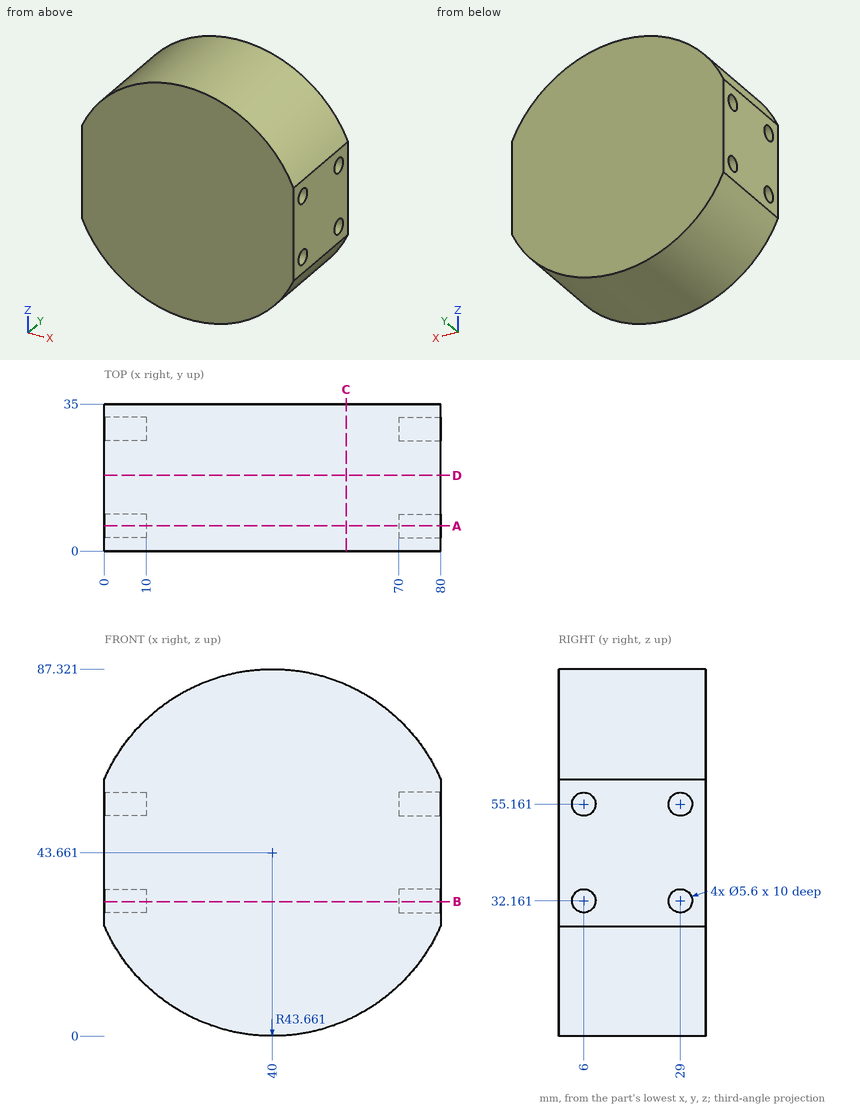
For this review, use the dimensioned drawing (mm, ordinates from the lowest corner) and the shaded views. Coordinates: 2 decimals unless noted, no trailing zeros. Order: outer loops, then holes, each group sorted by start corner. A loop starts at its lowest first (then second) coordinate and runs counter-clockwise, first axis right, second up. Notation, with made-up numbers: M 13,85 L 57,85 A13 ccw 57,105 Z; hole C 56,-13 d8. An arc over 180 degrees is marked long. Answer as a JSON object with one key per item and string values. Group by question number.
1) Add section B-B, the plane z = 32. Write out the cut boundary in (x, y) (1 decimal).
2) For pin 1 (5 mm diameter, centred on y = 6, z = 55.16, fed in from +X); pin 2 (6 mm diameter, centred on x = 68, y = 25, fed in from +Z) (1 decimal); pin 3 (2 mm diameter, centred on x = 59.5, y = 8.5, fed in from +Z), all flat-tipped, find the tip position at first contact; note any pin that passes through.
3) Add section D-D, the plane y = 18. Write out the cut boundary in (x, z), then the cut area to 3 significant figures.
4) Wall thickness on L1, parallel to Z at x = 8.5, y = 27 (1 decimal); L2, parallel to X at y = 19, z = 67; L3, parallel to Z at x = 59.5, y = 12 (1 decimal): over which ranges is each line inside the solid? List them lowest first.
5) Add section C-C, the plane x = 57.5. Write out the cut boundary in (y, z), then the cut area to 3 significant figures.
6) Add section A-A, the plane y = 6. Write out the cut boundary in (x, z).
Computed values:
{
 "1": {"outline": "M 0,0 L 80,0 L 80,3.2 L 70,3.2 L 70,8.8 L 80,8.8 L 80,26.2 L 70,26.2 L 70,31.8 L 80,31.8 L 80,35 L 0,35 L 0,31.8 L 10,31.8 L 10,26.2 L 0,26.2 L 0,8.8 L 10,8.8 L 10,3.2 L 0,3.2 Z"},
 "2": {"pin 1": "stops at x = 70", "pin 2": "stops at z = 79.5", "pin 3": "stops at z = 83.21"},
 "3": {"outline": "M 0,26.16 A43.66 ccw 80,26.16 L 80,61.16 A43.66 ccw 0,61.16 Z", "area": "5,820 mm^2"},
 "4": {"L1": "z = 13.4 to 30.2, 34.1 to 53.2, 57.1 to 73.9", "L2": "x = 3.1 to 76.9", "L3": "z = 4.6 to 82.7"},
 "5": {"outline": "M 0,3.66 L 35,3.66 L 35,83.66 L 0,83.66 Z", "area": "2,800 mm^2"},
 "6": {"outline": "M 0,26.16 A43.66 ccw 80,26.16 L 80,29.36 L 70,29.36 L 70,34.96 L 80,34.96 L 80,52.36 L 70,52.36 L 70,57.96 L 80,57.96 L 80,61.16 A43.66 ccw 0,61.16 L 0,57.96 L 10,57.96 L 10,52.36 L 0,52.36 L 0,34.96 L 10,34.96 L 10,29.36 L 0,29.36 Z"}
}
